Model file for the job. Use its own axes, mm. A direction names the side the tool comes from. Coordinates: 2 decimals unless noted, no trailing zeros. Write each loop counter-clockwise with the first axis right and the second up, starting at its lowest first coordinate (ties: lowest second). Pieces come first, ordered by that corner, then holes.
Q1. Drill centre lines: probe 1 along Z at (x, y) = (0, 2); probe 2 along X at (y, z) = (16, -14); probe 3 along X at (y, z) = (2.4, 38.1). Where is each one in solid material? Low to high.
Q2. Band-saw the part on D-D, the plane z = 45.5. Write the cut outline in (x, y), plus the area to 3 significant figures.
Q3. Pin check, flat tips, straight feed: P1, Ø1.5, axis at x = -14, z = 25, coming from the -Y side; P2, Ø15, axis at x = -2, z = -8.5, coming from the +Y side; P3, Ø6.5, axis at x = 0, z = -38.1, coming from the +Y side. Stop position of each tip, or through.
Q4. Band-saw the part on A-A, the plane x = 0. Write the cut outline in (y, z).
Q5. Which spindle directions (+Z, -Z, +X, -X, +Y, -Y) get a long thin tool onto all of the face, cutting with end or side? Do faces 4 (the cylindrical face through (-1.37, 2.16, -18.03)), 5 (the flat face through (-15.081, 16, 1)). Say none if no direction does.
Q6. Band-saw the part on B-B, the plane y = 21.25. Write the cut outline in (x, z), plus the area to 3 significant figures.
Q7. Pull direction Z, two halves, no side cores. Call faces 1 (the flat face through (0, 4, -57.15)), 2 (the flat face through (0, 6.35, 1)), 3 (the cylindrical face through (17.496, 11.003, -51.693)): released by +Z, released by -Z, zero draft, split by the parting line, or undercut.
Q8. Band-saw the part on C-C, the plane z = -38.1. Write the cut outline in (x, y), plus the area to 3 significant figures.
from build123d import *

# Parameters (mm, degrees)
BOSS_EXTRUDE1_DEPTH                                = 57.15
CSK_FOR_10_FLAT_HEAD_MACHINE_SCREW_100_D           = 5.1054
CSK_FOR_10_FLAT_HEAD_MACHINE_SCREW_100_CSINK_D     = 9.779
CSK_FOR_10_FLAT_HEAD_MACHINE_SCREW_100_CSINK_ANGLE = 100
SKETCH6_OUTSIDE_W                                  = 141.026
SKETCH6_OUTSIDE_H                                  = 52.126
SKETCH6_OUTSIDE_W_2                                = 114.3
SKETCH6_OUTSIDE_H_2                                = 25.4
SKETCH6_OUTSIDE_R                                  = 4.1671875
CUT_EXTRUDE2_DEPTH                                 = 75.070102985


with BuildPart() as part:
    # Sketch1 → Boss-Extrude1 (new, symmetric)
    with BuildSketch(Plane.XY):
        Polygon((-19.84375, 25.4), (-19.84375, 0), (19.84375, 0), (19.84375, 25.4), (15.08125, 25.4), (15.08125, 6.35), (-15.08125, 6.35), (-15.08125, 25.4), align=None)
    extrude(amount=BOSS_EXTRUDE1_DEPTH, both=True)

    # CSK for #10 Flat Head Machine Screw (100)1 (through all)
    with Locations(Plane(origin=(0, 6.35, 0), x_dir=(1, 0, 0), z_dir=(0, 1, 0))):
        with Locations((0, 15.875), (0, 38.1), (0, -15.875), (0, -38.1)):
            CounterSinkHole(CSK_FOR_10_FLAT_HEAD_MACHINE_SCREW_100_D / 2, CSK_FOR_10_FLAT_HEAD_MACHINE_SCREW_100_CSINK_D / 2, counter_sink_angle=CSK_FOR_10_FLAT_HEAD_MACHINE_SCREW_100_CSINK_ANGLE)

    # Sketch6 outside → Cut-Extrude2 (cut, through all)
    # profile 1 of 3: a face of its own
    with BuildSketch(Plane(origin=(19.84375, 0, 0), x_dir=(0, 0, -1), z_dir=(1, 0, 0))):
        with Locations((0, 12.7)):
            Rectangle(SKETCH6_OUTSIDE_W, SKETCH6_OUTSIDE_H)
        with Locations((0, 12.7)):
            Rectangle(SKETCH6_OUTSIDE_W_2, SKETCH6_OUTSIDE_H_2, mode=Mode.SUBTRACT)
    # profile 2 of 3: a face of its own
    with BuildSketch(Plane(origin=(19.84375, 0, 0), x_dir=(0, 0, -1), z_dir=(1, 0, 0))):
        with Locations(Location((-47.625, 11.90625, 0), (0, 0, 90))):
            Circle(SKETCH6_OUTSIDE_R)
    # profile 3 of 3: a face of its own
    with BuildSketch(Plane(origin=(19.84375, 0, 0), x_dir=(0, 0, -1), z_dir=(1, 0, 0))):
        with Locations(Location((47.625, 11.90625, 0), (0, 0, 90))):
            Circle(SKETCH6_OUTSIDE_R)
    extrude(amount=-CUT_EXTRUDE2_DEPTH, mode=Mode.SUBTRACT)


solid = part.part
Answer sheet:
1. probe 1: z = -57.15 to -40.65, -35.55 to -18.43, -13.32 to 13.32, 18.43 to 35.55, 40.65 to 57.15
1. probe 2: x = -19.84 to -15.08, 15.08 to 19.84
1. probe 3: x = -19.84 to -2.55, 2.55 to 19.84
2. outline: (-19.84, 0) - (19.84, 0) - (19.84, 8.32) - (15.08, 8.32) - (15.08, 6.35) - (-15.08, 6.35) - (-15.08, 8.32) - (-19.84, 8.32) - close; (-19.84, 15.49) - (-15.08, 15.49) - (-15.08, 25.4) - (-19.84, 25.4) - close; (15.08, 15.49) - (19.84, 15.49) - (19.84, 25.4) - (15.08, 25.4) - close
2. area: 365 mm2
3. P1: stops at y = 0
3. P2: stops at y = 6.35
3. P3: stops at y = 4.97
4. outline: (0, -57.15) - (6.35, -57.15) - (6.35, -42.99) - (4.39, -40.65) - (0, -40.65) - close; (0, -35.55) - (4.39, -35.55) - (6.35, -33.21) - (6.35, -20.76) - (4.39, -18.43) - (0, -18.43) - close; (0, -13.32) - (4.39, -13.32) - (6.35, -10.99) - (6.35, 10.99) - (4.39, 13.32) - (0, 13.32) - close; (0, 18.43) - (4.39, 18.43) - (6.35, 20.76) - (6.35, 33.21) - (4.39, 35.55) - (0, 35.55) - close; (0, 40.65) - (4.39, 40.65) - (6.35, 42.99) - (6.35, 57.15) - (0, 57.15) - close
5. face 4: +Y, -Y
5. face 5: +Z, -Z, +Y
6. outline: (-19.84, -57.15) - (-15.08, -57.15) - (-15.08, 57.15) - (-19.84, 57.15) - close; (15.08, -57.15) - (19.84, -57.15) - (19.84, 57.15) - (15.08, 57.15) - close
6. area: 1,090 mm2
7. face 1: released by -Z
7. face 2: zero draft
7. face 3: undercut
8. outline: (-19.84, 0) - (-2.55, 0) - (-2.55, 4.39) - (-4.89, 6.35) - (-15.08, 6.35) - (-15.08, 25.4) - (-19.84, 25.4) - close; (2.55, 0) - (19.84, 0) - (19.84, 25.4) - (15.08, 25.4) - (15.08, 6.35) - (4.89, 6.35) - (2.55, 4.39) - close
8. area: 396 mm2
